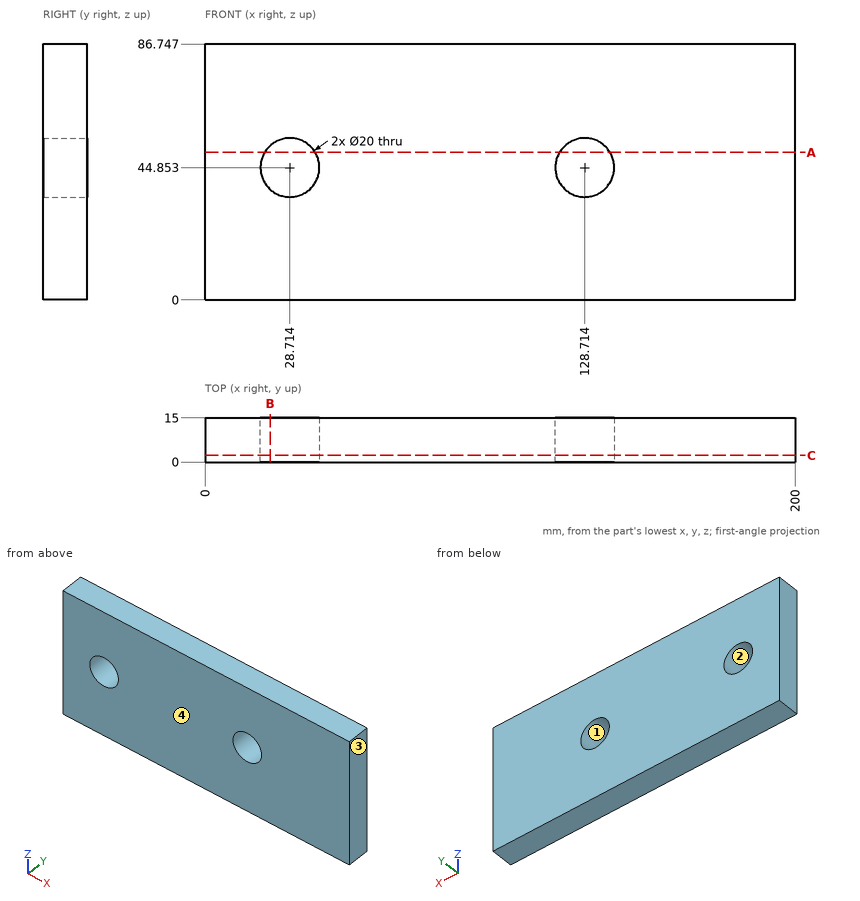
Geometry check sheet. Reference: drawing and pictorial views, mm from the part's lowest x, y, z. Coordinates: 2 decimals unless noted, no trailing zeros. Write each loop counter-clockwise with the first axis right and the second up, starting at its lowest first coordinate (ties: lowest second). Pieces come first, ordered by that corner, then holes. Notation, with made-up numbers: M 8,29.25 L 37,29.25 A16 ccw 37,37.25 Z; hole C 13,59.25 d11. An arc over 180 degrees is marked long. Write item = value, one per line. Start each with the question number.
1. Sectioned sample at B-B (x = 22). Record the cut outline in (y, z).
2. Sectioned sample at A-A (z = 50). Record the cut outline in (x, y), then the cut area to 3 significant figures.
3. Mould release check, pull along X, two halves, no side actions. Record for the marked faces 1, 2, 3 and 4: pulls with the +X half, pulls with the -X half, needs draft (parallel to the pull), parting line crosses it, or undercut.
4. Sectioned sample at C-C (y = 2.25). Record the cut outline in (x, z).
5. Thickness scan on probe 1 along X at (y, z) = (10.75, 46); probe 2 along X at (y, z) = (7.25, 42); probe 3 along Z at (x, y) = (129.5, 6). Record the ranges inside material, lowest first.
The answers:
q1.outline = M 0,0 L 15,0 L 15,37.44 L 0,37.44 Z; M 0,52.26 L 15,52.26 L 15,86.75 L 0,86.75 Z
q2.outline = M 0,0 L 20.14,0 L 20.14,15 L 0,15 Z; M 37.29,0 L 120.14,0 L 120.14,15 L 37.29,15 Z; M 137.29,0 L 200,0 L 200,15 L 137.29,15 Z
q2.area = 2,490 mm²
q3.face_1 = undercut
q3.face_2 = undercut
q3.face_3 = pulls with the +X half
q3.face_4 = needs draft
q4.outline = M 0,0 L 200,0 L 200,86.75 L 0,86.75 Z; hole C 28.71,44.85 d20; hole C 128.71,44.85 d20
q5.probe_1 = 0 to 18.78, 38.65 to 118.78, 138.65 to 200
q5.probe_2 = 0 to 19.13, 38.3 to 119.13, 138.3 to 200
q5.probe_3 = 0 to 34.88, 54.82 to 86.75
